Study the drawing (mm; zero at the part's minimum x, y, z) and answer. Coordinates: 2 decimals unless noted, no trailing zeros. Write each loop counter-clockwise with the first axis right and the second up, starting at its lowest first coordinate (ties: lowest second). Pieces come first, ordered by that corner, then holes. Notation, with made-up numbers: M 40.25,65 L 77.25,65 A15 cw 77.25,78 Z; hole C 79.25,6.5 d8. An arc over 180 degrees is marked long. Answer as a JSON object with one key per item and string values. Group by question number.
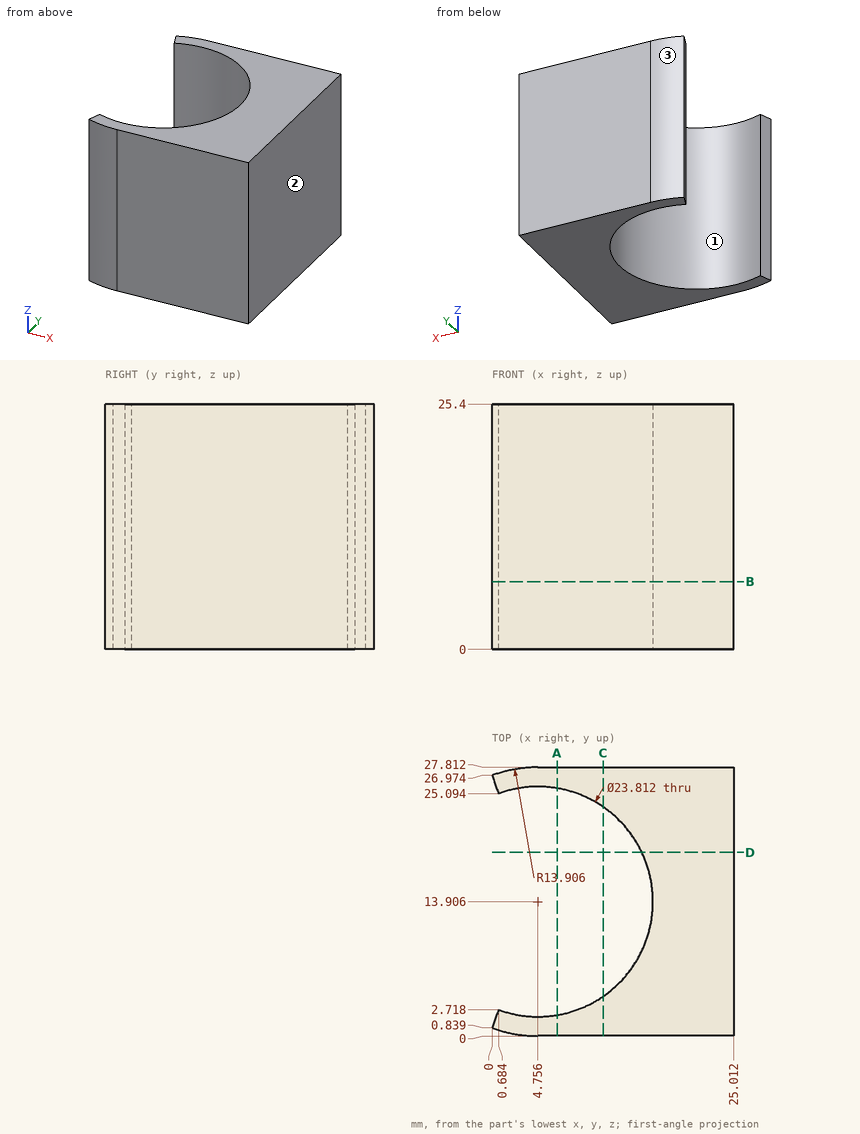
Item 1: A cutting plane is placed at A-A, the plane x = 6.75. Write down the section's boundary in (y, z) (1 decimal).
Item 2: Flat-ended cylindrical pins translate along their axes: pin 1 Ø2 at (y, z) = (6, 4) entering from -X; pin 2 Ø6 at (y, z) = (19, 20.5) entering from -X. Find the tip coordinate at first contact, or state that the pin passes through.
Item 3: Consider L1, parallel to Y at x = 15.75, z = 20.5 (1 decimal); L2, parallel to Y at x = 4.5, z = 16; L3, parallel to X at y = 14, z = 17.75. Determine where each line is inside the solid, lowest interval first. Write a range as from..to.
Item 4: A cutting plane is placed at D-D, the plane y = 19. Write down the section's boundary in (x, z), and give its area (3 significant figures).
Item 5: For a pull along X with two mould halves and no side action, classify the marked faces 1, 2 and 3 as +X half, -X half, draft (parallel to the pull), parting line (faces both ways), or undercut.
Item 6: A cutting plane is placed at C-C, the plane x = 11.5. Write down the section's boundary in (y, z), and give its area (3 significant figures).
Item 7: A cutting plane is placed at B-B, the plane z = 7. Write down the section's boundary in (x, y) (1 decimal).
Answer:
{
 "1": {"outline": "M 0,0 L 2.2,0 L 2.2,25.4 L 0,25.4 Z; M 25.6,0 L 27.8,0 L 27.8,25.4 L 25.6,25.4 Z"},
 "2": {"pin 1": "x = 12.66", "pin 2": "x = 13.49"},
 "3": {"L1": "0..9.3, 18.5..27.8", "L2": "0..2, 25.81..27.81", "L3": "16.66..25.01"},
 "4": {"outline": "M 15.52,0 L 25.01,0 L 25.01,25.4 L 15.52,25.4 Z", "area": "241 mm2"},
 "5": {"face 1": "undercut", "face 2": "+X half", "face 3": "-X half"},
 "6": {"outline": "M 0,0 L 4.09,0 L 4.09,25.4 L 0,25.4 Z; M 23.72,0 L 27.81,0 L 27.81,25.4 L 23.72,25.4 Z", "area": "208 mm2"},
 "7": {"outline": "M 0,0.8 A13.9 ccw 4.8,0 L 25,0 L 25,27.8 L 4.8,27.8 A13.9 ccw 0,27 L 0.7,25.1 A11.9 cw long 0.7,2.7 Z"}
}
